For this review, take the finished solid that the model builds, in its own axes (mm). A direction names the side the tool comes from. Give positions to 0.01 mm unless a question says otherwise; leave off trailing zeros. Order: outer loops, then holes, each group sorted by start corner. A loop starts at its lowest first (then second) coordinate and runs counter-clockwise, first axis right, second up. Notation, with made-up numbers: (80.25, 88) - (132.25, 88) arc R22 cw to (132.25, 124) - close; hole circle Ø7 at (1.25, -8.5). An arc over 180 degrees is marked (long way). Put each result on its own line as item: value. Start each with the question number.
```python
from build123d import *

# Parameters (mm, degrees)
SKETCH2_W           = 60
SKETCH2_H           = 20
SKETCH2_W_2         = 10
SKETCH2_H_2         = 9.423036009
BOSS_EXTRUDE1_DEPTH = 5
BOSS_EXTRUDE2_DEPTH = 30


with BuildPart() as part:
    # Sketch2 → Boss-Extrude1 (new body)
    with BuildSketch(Plane(origin=(0, 0, 0), x_dir=(1, 0, 0), z_dir=(0, 1, 0))):
        Rectangle(SKETCH2_W, SKETCH2_H)
        with Locations((0, 14.711518005)):
            Rectangle(SKETCH2_W_2, SKETCH2_H_2)
    extrude(amount=BOSS_EXTRUDE1_DEPTH)

    # Sketch2_3 → Boss-Extrude2 (add)
    with BuildSketch(Plane(origin=(0, 0, 0), x_dir=(1, 0, 0), z_dir=(0, 1, 0))):
        Polygon((-5, 19.423036009), (-5, 10), (0, 10), (5, 10), (5, 19.423036009), align=None)
    extrude(amount=-BOSS_EXTRUDE2_DEPTH)


solid = part.part
```
1. Add section A-A, the plane y = -18.5. Give the boundary of the cut face in (x, z), then the cut area to 3 significant figures.
2. Wall thickness on line 1 (Y direction, x = -8.5, z = 3); line 2 (Z direction, x = -11, y = 3); line 3 (X direction, y = -12, z = -13.5): over which ranges is each line inside the solid? List them lowest first. Write a range as from..to.
3. Clearance check with flat-ended pins moving along their axes: pin 1 (10.5 mm diameter, centred on y = -10, z = -14.5, fed in from +X); pin 2 (4.5 mm diameter, centred on y = -20.5, z = -13, fed in from -X); pin 3 (8 mm diameter, centred on x = -1.5, y = -11, fed in from +Z); pin 4 (2 mm diameter, centred on y = -10, z = -8, fed in from +X). State where each tip first meets the part, or that it passes through.
4. Add section B-B, the plane z = 4.25. Give the boundary of the cut face in (x, y), then the cut area to 3 significant figures.
5. Tool access review of faces 1 (the face through (0, -15, -10)), 2 (the face through (-18, 2, -10)), 3 (the face through (17, 2, -10)): name each direction out of +Z, -Z, +X, -X, +Y, -Y from which nothing blocks a thin tool from reaching the whole face with its end or side.
Found:
1. outline: (-5, -19.42) - (5, -19.42) - (5, -10) - (-5, -10) - close
1. area: 94.2 mm^2
2. line 1: y = 0..5
2. line 2: z = -10..10
2. line 3: x = -5..5
3. pin 1: stops at x = 5
3. pin 2: stops at x = -5
3. pin 3: stops at z = -10
3. pin 4: passes through
4. outline: (-30, 0) - (30, 0) - (30, 5) - (-30, 5) - close
4. area: 300 mm^2
5. face 1: +Z, +X, -X, -Y
5. face 2: -Z, -X, +Y, -Y
5. face 3: -Z, +X, +Y, -Y
